Part model, mm, in its own coordinate system. A direction names the side the tool comes from. Round coordinates to 2 decimals unless told otherwise and drop trailing zeros. Loops run counter-clockwise (first coordinate to the right, second up) from the corner with the lowest first, then second, coordinate; pieces in that order, holes last.
Autodesk Inventor part; units mm, degrees
ref_plane "YZ Plane" through (0, 0, 0) normal (1, 0, 0) x (0, 1, 0)
ref_plane "XZ Plane" through (0, 0, 0) normal (0, 1, 0) x (-1, 0, 0)
ref_plane "XY Plane" through (0, 0, 0) normal (0, 0, 1) x (1, 0, 0)
sketch "Sketch1" plane through (0, 0, 0) normal (0, 0, 1) x (1, 0, 0)
  line L0 (10, 0) -> (40, 0)
  line L1 (50, 10) -> (50, 29.4958)
  line L2 (40, 39.4958) -> (10, 39.4958)
  line L3 (0, 29.4958) -> (0, 10)
  arc A0 (10, 39.4958) -> (0, 29.4958) centre (10, 29.4958) ccw
  arc A1 (50, 29.4958) -> (40, 39.4958) centre (40, 29.4958) ccw
  arc A2 (40, 0) -> (50, 10) centre (40, 10) ccw
  arc A3 (0, 10) -> (10, 0) centre (10, 10) ccw
  point P0 (0, 0)
  point P1 (50, 39.4958)
  point P2 (0, 39.4958)
  dimension "d0" = 50
  dimension "d1" = 10
extrude "Extrusion1" add sketch "Sketch1" along normal blind 25
sketch "Sketch2" plane through (0, 0, 25) normal (0, 0, 1) x (1, 0, 0)
  line L0 (39.1979, 34.3605) -> (27.5461, 34.3605)
  line L1 (22.5461, 29.3605) -> (22.5461, 23.1687)
  line L2 (27.5461, 18.1687) -> (39.1979, 18.1687)
  line L3 (44.1979, 23.1687) -> (44.1979, 29.3605)
  arc A0 (27.5461, 34.3605) -> (22.5461, 29.3605) centre (27.5461, 29.3605) ccw
  arc A1 (44.1979, 29.3605) -> (39.1979, 34.3605) centre (39.1979, 29.3605) ccw
  arc A2 (39.1979, 18.1687) -> (44.1979, 23.1687) centre (39.1979, 23.1687) ccw
  arc A3 (22.5461, 23.1687) -> (27.5461, 18.1687) centre (27.5461, 23.1687) ccw
  line L4 (27.5461, 31.9141) -> (39.1979, 31.9141)
  arc A4 (41.7515, 29.3605) -> (39.1979, 31.9141) centre (39.1979, 29.3605) ccw
  line L5 (41.7515, 29.3605) -> (41.7515, 23.1687)
  arc A5 (39.1979, 20.6151) -> (41.7515, 23.1687) centre (39.1979, 23.1687) ccw
  line L6 (39.1979, 20.6151) -> (27.5461, 20.6151)
  arc A6 (24.9925, 23.1687) -> (27.5461, 20.6151) centre (27.5461, 23.1687) ccw
  line L7 (24.9925, 23.1687) -> (24.9925, 29.3605)
  arc A7 (27.5461, 31.9141) -> (24.9925, 29.3605) centre (27.5461, 29.3605) ccw
  circle A8 centre (35.2717, 26.2646) radius 4.2058
  point P0 (0, 0)
  dimension "d4" = 5
extrude "Extrusion2" add sketch "Sketch2" along normal blind 3
fillet "Fillet1" radius 3 1 edges at (31.0659, 26.2646, 28)
sketch "Sketch3" plane through (10, 0, 0) normal (0, -1, 0) x (1, 0, 0)
  circle A0 centre (14.5059, 11.6029) radius 2.3072
  point P0 (-10, 0)
extrude "Extrusion3" add sketch "Sketch3" along normal blind 1
properties part number "temp camera" material "Rubber"
1) Slice it at B-B, the plane x = 30. Give the cut face in (y, z), then the cut area to 3 significant figures.
Values:
outline: (0, 0) - (39.5, 0) - (39.5, 25) - (34.36, 25) - (34.36, 28) - (31.91, 28) - (31.91, 25) - (20.62, 25) - (20.62, 28) - (18.17, 28) - (18.17, 25) - (0, 25) - close
area: 1,000 mm2
2) Wall check: line 1 along Y through (x, z) = (14.5, 10.5); line 2 along Z through (x, y) = (18.5, 10); line 3 along X through (y, z) = (6, 20.75). Give the ranges that are in metal, low to high.
Values:
line 1: y = 0 to 39.5
line 2: z = 0 to 25
line 3: x = 0.83 to 49.17
3) Slice it at D-D, the plane x = 15.5. Give the cut face in (y, z), then the cut area to 3 significant figures.
Values:
outline: (0, 0) - (39.5, 0) - (39.5, 25) - (0, 25) - close
area: 987 mm2
4) Slice it at A-A, the plane z = 16.5. Give the cut face in (x, y), then the cut area to 3 significant figures.
Values:
outline: (0, 10) arc R10 ccw to (10, 0) - (40, 0) arc R10 ccw to (50, 10) - (50, 29.5) arc R10 ccw to (40, 39.5) - (10, 39.5) arc R10 ccw to (0, 29.5) - close
area: 1,890 mm2
5) Tool access for faces 1 (the face through (42.8, 19.7, 26.5)), 2 (the face through (33, 34.36, 26)), 3 (the face through (41.752, 26, 26)), 4 (the face through (33, 18.169, 26)): list every direction of +Z, -Z, +X, -X, +Y, -Y with a clear straight run to the whole face (end or side of a thin tool).
Values:
face 1: +Z, +X, -Y
face 2: +Z, +X, -X, +Y
face 3: +Z
face 4: +Z, +X, -X, -Y
6) Slice it at C-C, the plane y = 13. Give the cut face in (x, z).
Values:
outline: (0, 0) - (50, 0) - (50, 25) - (0, 25) - close
7) Drop flat-ended pins along their axis: pin 1 Ø0.9 at (y, z) = (25, 26.5) entering from -X; pin 2 Ø10 at (x, y) = (17, 11) entering from +Z; pin 3 Ø10 at (x, z) = (12.5, 6.5) entering from -Y. Give the stop position or say it passes through.
Values:
pin 1: stops at x = 22.55
pin 2: stops at z = 25
pin 3: stops at y = 0
8) Mould opens along X. For faces 5 (the face through (22.546, 26, 26)), 6 (the face through (33, 31.914, 26)), 7 (the face through (35, 26, 28)) say: released by +X, released by -X, zero draft, split by the parting line, or undercut.
Values:
face 5: released by -X
face 6: undercut
face 7: zero draft
